from build123d import *

# Parameters (mm, degrees)
F1_DEPTH = 2.4
F1_TAPER = 5
F3_DEPTH = 3
F4_R     = 10
F5_SIZE  = 0.5


with BuildPart() as f1:
    # F0 (on Top) → F1 (new body)
    with BuildSketch(Plane.XY):
        with BuildLine():
            Line((3.897114317, 3.55), (-3.897114317, 3.55))
            ThreePointArc((-3.897114317, 3.55), (-5.0229473419, 2.9), (-5.0229473419, 1.6))
            Line((-5.0229473419, 1.6), (-1.1258330249, -5.15))
            ThreePointArc((-1.1258330249, -5.15), (0, -5.8), (1.1258330249, -5.15))
            Line((1.1258330249, -5.15), (5.0229473419, 1.6))
            ThreePointArc((5.0229473419, 1.6), (5.0229473419, 2.9), (3.897114317, 3.55))
        make_face()
    extrude(amount=F1_DEPTH, taper=F1_TAPER)

    # F2 (on face) → F3 (join)
    with BuildSketch(Plane(origin=(0, 0, 0), x_dir=(1, 0, 0), z_dir=(0, 0, -1))):
        with BuildLine():
            Line((-15.7575166744, 6.788205417), (-5.8889727457, -3.4))
            Line((-5.8889727457, -3.4), (-2, -17.040512449))
            ThreePointArc((-2, -17.040512449), (0, -18.55), (2, -17.040512449))
            Line((2, -17.040512449), (5.8889727457, -3.4))
            Line((5.8889727457, -3.4), (15.7575166744, 6.788205417))
            ThreePointArc((15.7575166744, 6.788205417), (16.0647712402, 9.275), (13.7575166744, 10.2523070321))
            Line((13.7575166744, 10.2523070321), (0, 6.8))
            Line((0, 6.8), (-13.7575166744, 10.2523070321))
            ThreePointArc((-13.7575166744, 10.2523070321), (-16.0647712402, 9.275), (-15.7575166744, 6.788205417))
        make_face()
    extrude(amount=F3_DEPTH)

    # F4
    f4_edges = [f1.edges().sort_by_distance(p)[0] for p in [
        (0, -6.8, -1.5),
        (5.888973, 3.4, -1.5),
        (-5.888973, 3.4, -1.5),
    ]]
    fillet(f4_edges, radius=F4_R)

    # F5
    f5_edges = [f1.edges().sort_by_distance(p)[0] for p in [
        (-11.696199, -2.595334, -3),
        (-6.157481, 3.555024, -3),
        (-16.064771, -9.275, -3),
        (-3.600474, 11.426873, -3),
        (-8.095725, -8.831539, -3),
        (0, 18.55, -3),
        (0, -7.110047, -3),
        (3.600474, 11.426873, -3),
        (8.095725, -8.831539, -3),
        (6.157481, 3.555024, -3),
        (16.064771, -9.275, -3),
        (11.696199, -2.595334, -3),
    ]]
    chamfer(f5_edges, length=F5_SIZE)


solid = f1.part
Verification items for the finished model (mm, model axes). A direction names the side the tool comes from. Give positions to 0.01 mm unless a question says otherwise; leave off trailing zeros. Write each loop counter-clockwise with the first axis right and the second up, starting at its lowest first coordinate (ties: lowest second). Pieces come first, ordered by that corner, then holes. Notation, with made-up numbers: M 5,63.5 L 33,63.5 A10 ccw 33,67.5 Z; hole C 4,39.25 d6. An arc over 180 degrees is marked long. Put each result on its own line as item: value. Start each with the question number.
1. Scan lines: line 1 along Z through (x, y) = (-12, -4); line 2 along X through (y, z) = (-5.25, 1); line 3 along X through (y, z) = (14.75, -2.25). Record each from-to range of solid material in increasing order. Write a range as [from, to].
2. Go/stop test with a flat-tipped pin: pin 1 Ø1.5 at (x, z) = (10.5, -0.5) entering from +Y. Record where the tip stops, or that it passes through.
3. Section check D-D (z = 1.3). Record the cut outline in (x, y).
4. Draft check along X on faces 4 (the face through (-0.03, -7.11, -1.27)), 5 (the face through (-0.04, 18.55, -1.23)), 6 (the face through (5.969, 3.486, -2.698)). Enter one of: +X half, -X half, draft (parallel to the pull), parting line (faces both ways), or undercut.
5. Section check B-B (y = -1.25). Record the cut outline in (x, z).
6. Section check A-A (z = -1.2). Record the cut outline in (x, y).
7. Set-up check for faces 1 (the face through (8.24, -8.61, -2.75)), 2 (the face through (11.46, -2.71, -2.75)), 3 (the face through (0, 4, 0)): record each of +Z, -Z, +X, -X, +Y, -Y from which the full face is reachable in a straight line by a thin tool's end or side.
8. Section check C-C (x = 10). Record the cut outline in (y, z).
Answer list:
1. line 1: [-3, 0]
1. line 2: [-0.95, 0.95]
1. line 3: [-2.65, 2.65]
2. pin 1: y = -0.59
3. outline: M -4.92,1.66 L -1.03,-5.09 A1.19 ccw 1.03,-5.09 L 4.92,1.66 A1.19 ccw 3.9,3.44 L -3.9,3.44 A1.19 ccw Z
4. face 4: undercut
4. face 5: parting line
4. face 6: +X half
5. outline: M -10.39,-2.5 L -9.7,-3 L 9.7,-3 L 10.39,-2.5 L 10.39,0 L 3.38,0 L 3.14,2.4 L -3.14,2.4 L -3.38,0 L -10.39,0 Z
6. outline: M -15.76,-6.79 A2.08 ccw -13.76,-10.25 L -2.43,-7.41 A10 cw 2.43,-7.41 L 13.76,-10.25 A2.08 ccw 15.76,-6.79 L 7.63,1.6 A10 cw 5.2,5.81 L 2,17.04 A2.08 ccw -2,17.04 L -5.2,5.81 A10 cw -7.63,1.6 Z
7. face 1: -Z, -Y
7. face 2: -Z, +X, +Y
7. face 3: +Z
8. outline: M -9.31,-2.5 L -8.79,-3 L -1.56,-3 L -0.84,-2.5 L -0.84,0 L -9.31,0 Z
